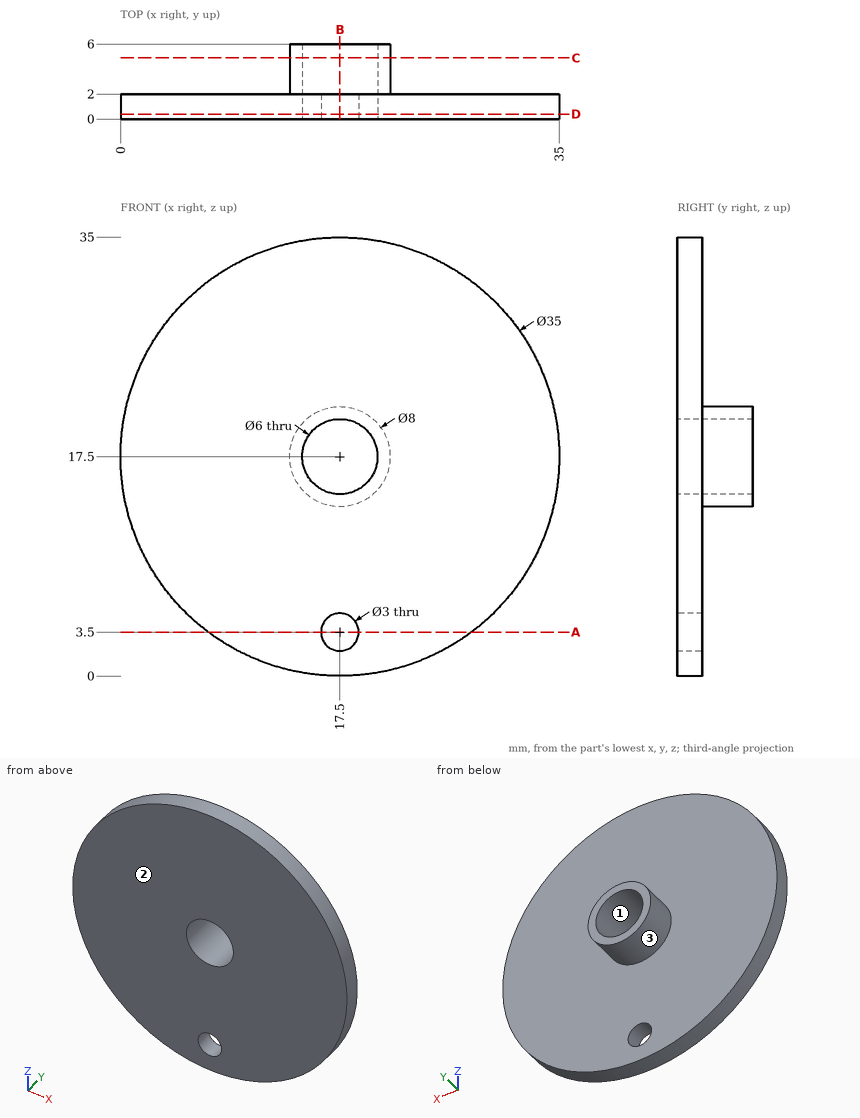
Answer from the drawing. Dimensions are ordinates in mm from the lowest x, y and z of the part. Round coordinates to 2 decimals unless told otherwise and drop trailing zeros. Write each loop counter-clockwise with the first axis right and the second up, starting at its lowest first coordinate (ties: lowest second). Pieces come first, ordered by that corner, then holes. Notation, with made-up numbers: (58, -11.5) - (84, -11.5) arc R26 cw to (84, 15.5) - close; hole circle Ø3 at (8.5, 11.25). An arc over 180 degrees is marked (long way). Use a Markdown table: item, result.
(1) The part is cut by section D-D (y = 0.4). Write down the section's boundary in (x, z), then the cut area to 3 significant figures.
Reported:
| item | result |
|---|---|
| outline | circle Ø35 at (17.5, 17.5); hole circle Ø6 at (17.5, 17.5); hole circle Ø3 at (17.5, 3.5) |
| area | 927 mm2 |
(2) The part is cut by section C-C (y = 4.9). Write down the section's boundary in (x, z), then the cut area to 3 significant figures.
Reported:
| item | result |
|---|---|
| outline | circle Ø8 at (17.5, 17.5); hole circle Ø6 at (17.5, 17.5) |
| area | 22.0 mm2 |
(3) The part is cut by section B-B (x = 17.5). Write down the section's boundary in (y, z), then the cut area to 3 significant figures.
Reported:
| item | result |
|---|---|
| outline | (0, 0) - (2, 0) - (2, 2) - (0, 2) - close; (0, 5) - (2, 5) - (2, 13.5) - (6, 13.5) - (6, 14.5) - (0, 14.5) - close; (0, 20.5) - (6, 20.5) - (6, 21.5) - (2, 21.5) - (2, 35) - (0, 35) - close |
| area | 60.0 mm2 |
(4) The mould has two halves that part along Z. Classify the marked faces 1, 2 and 3: released by +Z, released by -Z, zero draft, split by the parting line, or undercut.
Reported:
| item | result |
|---|---|
| face 1 | undercut |
| face 2 | zero draft |
| face 3 | split by the parting line |
(5) Straight lines are drawn through the part: line 1 along X through (y, z) = (1.6, 17.5); line 2 along X through (y, z) = (4.2, 17.5); line 3 along Y through (x, z) = (12, 25). For each, find the intervals that lie inside material, in ascending order. Write a range as [from, to].
Reported:
| item | result |
|---|---|
| line 1 | [0, 14.5], [20.5, 35] |
| line 2 | [13.5, 14.5], [20.5, 21.5] |
| line 3 | [0, 2] |
(6) Each of these flat-tipped pins is pushed along its axis until it touches: pin 1 Ø1 at (y, z) = (3.5, 14.5) entering from +X; pin 2 Ø6 at (x, z) = (24, 30.5) entering from +Y. Where does it stop, or does it pass through?
Reported:
| item | result |
|---|---|
| pin 1 | x = 20.62 |
| pin 2 | y = 2 |
(7) The part is cut by section A-A (z = 3.5). Write down the section's boundary in (x, y).
Reported:
| item | result |
|---|---|
| outline | (7, 0) - (16, 0) - (16, 2) - (7, 2) - close; (19, 0) - (28, 0) - (28, 2) - (19, 2) - close |
